```python
from build123d import *

# Parameters (mm, degrees)
F1_DEPTH = 30
F2_R     = 14.99999
F4_DEPTH = 20


# Not quite as in the source:
# - a fillet or chamfer is up to 0.001 mm smaller than in the source, because OpenCascade refuses the exact size


with BuildPart() as f1:
    # F0 (on Top) → F1 (new body)
    with BuildSketch(Plane.XY):
        Polygon((0, 40), (0, 0), (60, 0), (60, 10), (30, 10), (30, 30), (20, 30), (20, 40), align=None)
    extrude(amount=F1_DEPTH)

    # F2 (radius 15 in the source; OpenCascade refuses exactly that, so slightly less here)
    f2_edges = [f1.edges().sort_by_distance(p)[0] for p in [
        (0, 20, 30),
        (0, 20, 0),
    ]]
    fillet(f2_edges, radius=F2_R)

    # F3 (on face) → F4 (join)
    with BuildSketch(Plane(origin=(0, 10, 0), x_dir=(-1, 0, 0), z_dir=(0, 1, 0))):
        Polygon((-30, 0), (-30, 30), (-45, 0), align=None)
    extrude(amount=F4_DEPTH)


solid = f1.part
```
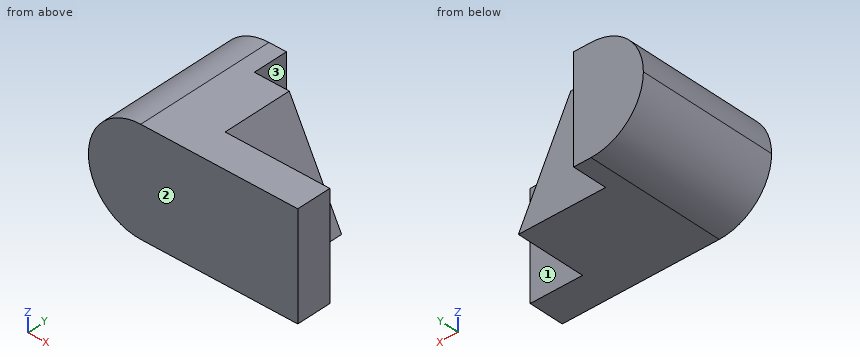
Read the model definition and answer for the solid it produces. Units are mm, in the model's axes. Face numbers are marked on the shaded views. A direction names the side the tool comes from. Give positions to 0.01 mm unless a question says otherwise; leave off trailing zeros. Write each loop counter-clockwise with the first axis right and the second up, starting at its lowest first coordinate (ties: lowest second). Pieces come first, ordered by that corner, then holes. Notation, with made-up numbers: (-5, -35) -> (40, -35) arc R15 cw to (40, -28) -> close; hole circle Ø9 at (65.5, 6.5). An arc over 180 degrees is marked (long way). Answer in a Markdown table with one row per item.
1) Section B-B on z = 14 is taken. Give the vertices of the cut face in (x, y).
Results list:
| item | result |
|---|---|
| outline | (0.03, 0) -> (60, 0) -> (60, 10) -> (38, 10) -> (38, 30) -> (20, 30) -> (20, 40) -> (0.03, 40) -> close |
2) A tool of negligible diameter and unlimited length cuts with its end or side. For the marked faces 1, 2 and 3, from which of +Z, -Z, +X, -X, +Y, -Y can it reach the whole face along a straight path? Write none if from no direction.
Results list:
| item | result |
|---|---|
| face 1 | +Z, +X, +Y |
| face 2 | +Z, -Z, +X, -X, -Y |
| face 3 | +Z, -Z, +X, +Y |
3) Each of these flat-tipped pins is pushed along its axis until it touches: pin 1 Ø3 at (y, z) = (37.5, 22.5) entering from +X; pin 2 Ø1 at (y, z) = (33, 13) entering from -X; pin 3 Ø8 at (x, z) = (21.5, 10.5) entering from -Y; pin 4 Ø12.5 at (x, z) = (27.5, 14.5) entering from +Y. Where does it stop, or does it pass through?
Results list:
| item | result |
|---|---|
| pin 1 | x = 20 |
| pin 2 | x = 0.08 |
| pin 3 | y = 0 |
| pin 4 | y = 30 |
4) Straight lines are drawn through the part: line 1 (Y direction, x = 21.5, z = 15); line 2 (Y direction, x = 47, z = 3.5); line 3 (Z direction, x = 35, y = 11). For each, find the intervals that lie inside material, in ascending order. Write a range as [from, to].
Results list:
| item | result |
|---|---|
| line 1 | [0, 30] |
| line 2 | [0, 10] |
| line 3 | [0, 20] |
5) Section C-C on x = 56.5 is taken. Give the vertices of the cut face in (y, z).
Results list:
| item | result |
|---|---|
| outline | (0, 0) -> (10, 0) -> (10, 30) -> (0, 30) -> close |
